Verification items for this drawing (mm, ordinates from the low corner). A direction names the side the tool comes from. Coordinates: 2 decimals unless noted, no trailing zeros. Loops run counter-clockwise (first coordinate to the right, second up) from the corner with the lowest first, then second, coordinate; pieces in that order, holes last. Notation, with made-up numbers: (12, 47) - (19, 47) arc R8 ccw to (19, 57) - close; hole circle Ø10 at (44.25, 88.25). An arc over 180 degrees is marked (long way). One line per item, written item: value. Start each with the question number.
(1) Section check C-C (z = 19.5). Record the boundary of the cut face in (x, y), plus the area to 3 significant figures.
(2) Gauge pin test, flat ends, axial feed: P1, Ø3, axis at x = 24.5, y = 1.5, coming from the +Z side; P2, Ø6, axis at x = 4.5, z = 19.5, coming from the +Y side; P3, Ø4.5, axis at x = 3.5, z = 17.5, coming from the -Y side. Record the tip position at first contact, or that the pin passes through.
(3) Draft check along Z on the marked faces 1, 2, 3 and 4. Enter one of: +Z half, -Z half, draft (parallel to the pull), parting line (faces both ways), or undercut.
(4) Section check B-B (x = 4.5). Record the boundary of the cut face in (y, z), plus the area to 3 significant figures.
(5) Set-up check for the marked faces 5, 6 and 7: record each of +Z, -Z, +X, -X, +Y, -Y from which the full face is reachable in a straight line by a thin tool's end or side.
(6) Section check D-D (x = 21.25). Record the boundary of the cut face in (y, z).
(7) Section check A-A (y = 4). Record the boundary of the cut face in (x, z).
(8) Thickness scan on probe 1 along Z at (x, y) = (28.6, 4); probe 2 along Z at (x, y) = (4.5, 2.5); probe 3 along X at (y, z) = (4, 19.5). Record the ranges inside material, lowest first. Write a range as [from, to].
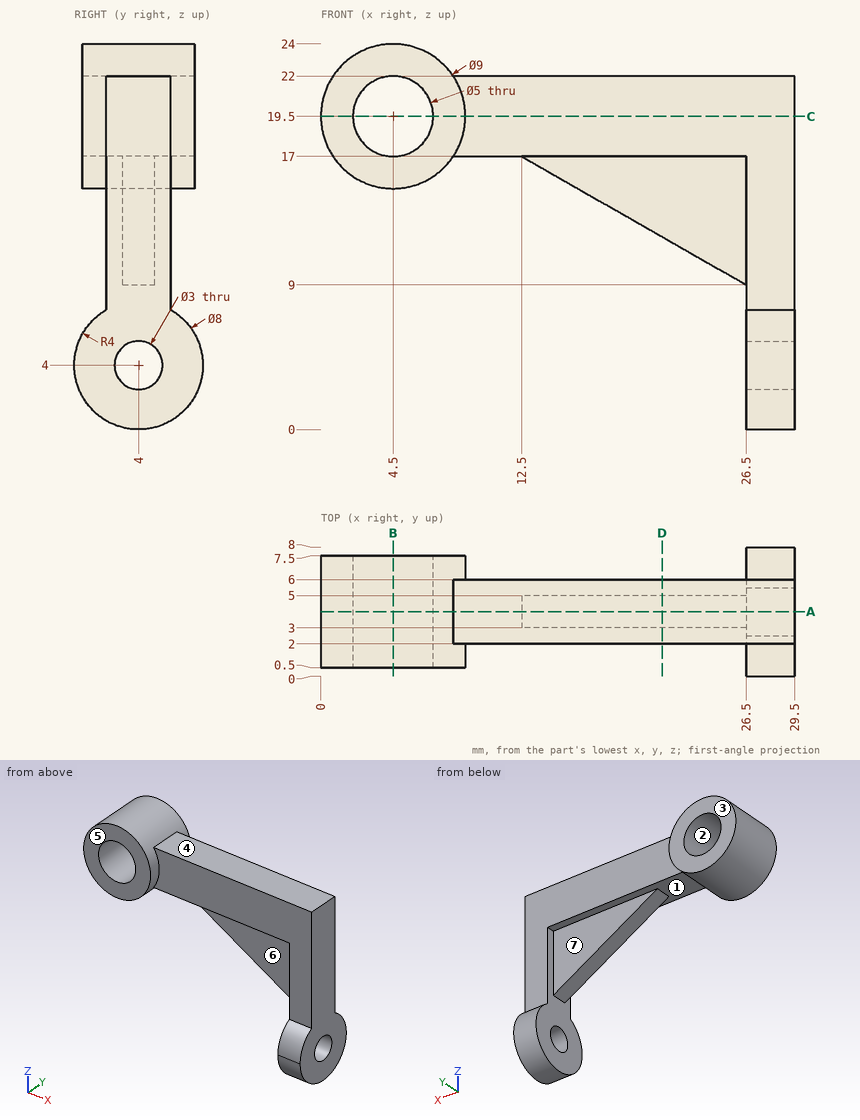
Responses:
1. outline: (0, 0.5) - (2, 0.5) - (2, 7.5) - (0, 7.5) - close; (7, 0.5) - (9, 0.5) - (9, 2) - (29.5, 2) - (29.5, 6) - (9, 6) - (9, 7.5) - (7, 7.5) - close
1. area: 110 mm²
2. P1: stops at z = 22
2. P2: stops at y = 7.5
2. P3: stops at y = 0.5
3. face 1: -Z half
3. face 2: undercut
3. face 3: draft
3. face 4: +Z half
4. outline: (0.5, 15) - (7.5, 15) - (7.5, 17) - (0.5, 17) - close; (0.5, 22) - (7.5, 22) - (7.5, 24) - (0.5, 24) - close
4. area: 28.0 mm²
5. face 5: +Z, -Z, +X, -X, -Y
5. face 6: -Z, -Y
5. face 7: -Z, +Y
6. outline: (2, 17) - (3, 17) - (3, 12) - (5, 12) - (5, 17) - (6, 17) - (6, 22) - (2, 22) - close
7. outline: (8.24, 17) - (12.5, 17) - (26.5, 9) - (26.5, 5.5) - (29.5, 5.5) - (29.5, 22) - (8.24, 22) arc R4.5 ccw (long way) to start; (26.5, 0) - (29.5, 0) - (29.5, 2.5) - (26.5, 2.5) - close; hole circle Ø5 at (4.5, 19.5)
8. probe 1: z = [0, 2.5], [5.5, 22]
8. probe 2: z = [15, 17], [22, 24]
8. probe 3: x = [0, 2], [7, 29.5]
